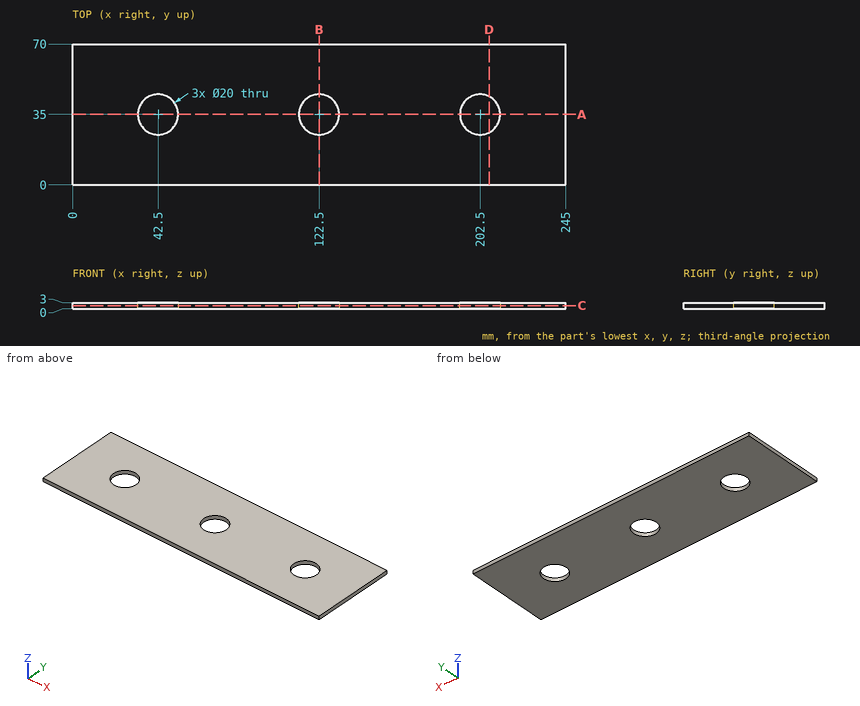
Answer from the drawing. Dimensions are ordinates in mm from the lowest x, y and z of the part. Round coordinates to 2 decimals unless told otherwise and drop trailing zeros. Write each loop counter-clockwise with the first axis right and the second up, starting at its lowest first coordinate (ties: lowest second). Pieces come first, ordered by that corner, then holes. Notation, with made-up numbers: M 34,31.5 L 85,31.5 A16 ccw 85,46.5 Z; hole C 78,9.5 d6. An arc over 180 degrees is marked long. Write each question's results on one line, items separated by ' | '. Start each with the question number.
Item 1: Find section D-D on x = 207. Write down the section's boundary in (y, z).
Item 2: Given pin 1 Ø18 at (x, y) = (42.5, 35) entering from -Z; pin 2 Ø1 at (x, z) = (124.5, 0.5) entering from -Y, each flat-ended and moving along its own axis, determine where each tip first touches the part or whether it passes through.
Item 3: Straight lines are drawn through the part: probe 1 along X at (y, z) = (34, 2.55); probe 2 along Y at (x, z) = (42.5, 0.65). For each, find the intervals that lie inside material, in ascending order.
Item 4: Find section C-C on z = 1.7. Write down the section's boundary in (x, y).
Item 5: Find section A-A on y = 35. Write down the section's boundary in (x, z).
Item 6: Find section B-B on x = 122.5. Write down the section's boundary in (y, z).
Answer block:
1) outline: M 0,0 L 26.07,0 L 26.07,3 L 0,3 Z; M 43.93,0 L 70,0 L 70,3 L 43.93,3 Z
2) pin 1: passes through | pin 2: stops at y = 0
3) probe 1: x = 0 to 32.55, 52.45 to 112.55, 132.45 to 192.55, 212.45 to 245 | probe 2: y = 0 to 25, 45 to 70
4) outline: M 0,0 L 245,0 L 245,70 L 0,70 Z; hole C 42.5,35 d20; hole C 122.5,35 d20; hole C 202.5,35 d20
5) outline: M 0,0 L 32.5,0 L 32.5,3 L 0,3 Z; M 52.5,0 L 112.5,0 L 112.5,3 L 52.5,3 Z; M 132.5,0 L 192.5,0 L 192.5,3 L 132.5,3 Z; M 212.5,0 L 245,0 L 245,3 L 212.5,3 Z
6) outline: M 0,0 L 25,0 L 25,3 L 0,3 Z; M 45,0 L 70,0 L 70,3 L 45,3 Z
